Could you check a few things on this model? Use its own coordinates, in mm. A direction names the side the tool comes from. Give positions to 0.01 mm unless a question says otherwise; leave off trailing zeros. Order: outer loops, then holes, each group sorted by start corner. A loop starts at its lowest first (then second) coordinate and runs counter-clockwise, first axis right, second up. Notation, with made-up numbers: (-22.75, 12) -> (25.25, 12) arc R31 ccw to (25.25, 49) -> close; hole circle Ø4 at (-7.75, 56.25). An arc over 180 degrees is marked (long way). One line per item, written item: value.
```python
from build123d import *

# Parameters (mm, degrees)
SKETCH_1_W          = 15.8
SKETCH_1_H          = 127.8
EXTRUDE_1_DEPTH     = 3.2
SKETCH_2_R          = 2.4
EXTRUDE_2_DEPTH     = 1.7
SKETCH_3_R          = 2.5
CUT_EXTRUDE_1_DEPTH = 1.8


with BuildPart() as part:
    # Эскиз1 → Бобышка-Вытянуть1 (new body)
    with BuildSketch(Plane.XY):
        Rectangle(SKETCH_1_W, SKETCH_1_H)
    extrude(amount=EXTRUDE_1_DEPTH)

    # Эскиз2 → Бобышка-Вытянуть2 (add)
    with BuildSketch(Plane.XY.offset(3.2)):
        with Locations(Location((-4, 60, 0), (0, 0, 180))):
            Circle(SKETCH_2_R)
        with Locations(Location((4, 60, 0), (0, 0, 180))):
            Circle(SKETCH_2_R)
        with Locations(Location((4, 52, 0), (0, 0, 180))):
            Circle(SKETCH_2_R)
        with Locations(Location((4, 44, 0), (0, 0, 180))):
            Circle(SKETCH_2_R)
        with Locations(Location((4, 36, 0), (0, 0, 180))):
            Circle(SKETCH_2_R)
        with Locations(Location((4, 28, 0), (0, 0, 180))):
            Circle(SKETCH_2_R)
        with Locations(Location((4, 20, 0), (0, 0, 180))):
            Circle(SKETCH_2_R)
        with Locations(Location((4, 12, 0), (0, 0, 180))):
            Circle(SKETCH_2_R)
        with Locations(Location((4, 4, 0), (0, 0, 180))):
            Circle(SKETCH_2_R)
        with Locations(Location((4, -4, 0), (0, 0, 180))):
            Circle(SKETCH_2_R)
        with Locations(Location((4, -12, 0), (0, 0, 180))):
            Circle(SKETCH_2_R)
        with Locations(Location((4, -20, 0), (0, 0, 180))):
            Circle(SKETCH_2_R)
        with Locations(Location((4, -28, 0), (0, 0, 180))):
            Circle(SKETCH_2_R)
        with Locations(Location((4, -36, 0), (0, 0, 180))):
            Circle(SKETCH_2_R)
        with Locations(Location((4, -44, 0), (0, 0, 180))):
            Circle(SKETCH_2_R)
        with Locations(Location((4, -52, 0), (0, 0, 180))):
            Circle(SKETCH_2_R)
        with Locations(Location((4, -60, 0), (0, 0, 180))):
            Circle(SKETCH_2_R)
        with Locations(Location((-4, 52, 0), (0, 0, 180))):
            Circle(SKETCH_2_R)
        with Locations(Location((-4, 44, 0), (0, 0, 180))):
            Circle(SKETCH_2_R)
        with Locations(Location((-4, 36, 0), (0, 0, 180))):
            Circle(SKETCH_2_R)
        with Locations(Location((-4, 28, 0), (0, 0, 180))):
            Circle(SKETCH_2_R)
        with Locations(Location((-4, 20, 0), (0, 0, 180))):
            Circle(SKETCH_2_R)
        with Locations(Location((-4, 12, 0), (0, 0, 180))):
            Circle(SKETCH_2_R)
        with Locations(Location((-4, 4, 0), (0, 0, 180))):
            Circle(SKETCH_2_R)
        with Locations(Location((-4, -4, 0), (0, 0, 180))):
            Circle(SKETCH_2_R)
        with Locations(Location((-4, -12, 0), (0, 0, 180))):
            Circle(SKETCH_2_R)
        with Locations(Location((-4, -20, 0), (0, 0, 180))):
            Circle(SKETCH_2_R)
        with Locations(Location((-4, -28, 0), (0, 0, 180))):
            Circle(SKETCH_2_R)
        with Locations(Location((-4, -36, 0), (0, 0, 180))):
            Circle(SKETCH_2_R)
        with Locations(Location((-4, -44, 0), (0, 0, 180))):
            Circle(SKETCH_2_R)
        with Locations(Location((-4, -52, 0), (0, 0, 180))):
            Circle(SKETCH_2_R)
        with Locations(Location((-4, -60, 0), (0, 0, 180))):
            Circle(SKETCH_2_R)
    extrude(amount=EXTRUDE_2_DEPTH)

    # Эскиз3 → Вырез-Вытянуть1 (cut)
    with BuildSketch(Plane(origin=(0, 0, 0), x_dir=(-1, 0, 0), z_dir=(0, 0, -1))):
        with Locations((-4, 60)):
            Circle(SKETCH_3_R)
        with Locations((4, 60)):
            Circle(SKETCH_3_R)
        with Locations((4, 52)):
            Circle(SKETCH_3_R)
        with Locations((4, 44)):
            Circle(SKETCH_3_R)
        with Locations((4, 36)):
            Circle(SKETCH_3_R)
        with Locations((4, 28)):
            Circle(SKETCH_3_R)
        with Locations((4, 20)):
            Circle(SKETCH_3_R)
        with Locations((4, 12)):
            Circle(SKETCH_3_R)
        with Locations((4, 4)):
            Circle(SKETCH_3_R)
        with Locations((4, -4)):
            Circle(SKETCH_3_R)
        with Locations((4, -12)):
            Circle(SKETCH_3_R)
        with Locations((4, -20)):
            Circle(SKETCH_3_R)
        with Locations((4, -28)):
            Circle(SKETCH_3_R)
        with Locations((4, -36)):
            Circle(SKETCH_3_R)
        with Locations((4, -44)):
            Circle(SKETCH_3_R)
        with Locations((4, -52)):
            Circle(SKETCH_3_R)
        with Locations((4, -60)):
            Circle(SKETCH_3_R)
        with Locations((-4, 52)):
            Circle(SKETCH_3_R)
        with Locations((-4, 44)):
            Circle(SKETCH_3_R)
        with Locations((-4, 36)):
            Circle(SKETCH_3_R)
        with Locations((-4, 28)):
            Circle(SKETCH_3_R)
        with Locations((-4, 20)):
            Circle(SKETCH_3_R)
        with Locations((-4, 12)):
            Circle(SKETCH_3_R)
        with Locations((-4, 4)):
            Circle(SKETCH_3_R)
        with Locations((-4, -4)):
            Circle(SKETCH_3_R)
        with Locations((-4, -12)):
            Circle(SKETCH_3_R)
        with Locations((-4, -20)):
            Circle(SKETCH_3_R)
        with Locations((-4, -28)):
            Circle(SKETCH_3_R)
        with Locations((-4, -36)):
            Circle(SKETCH_3_R)
        with Locations((-4, -44)):
            Circle(SKETCH_3_R)
        with Locations((-4, -52)):
            Circle(SKETCH_3_R)
        with Locations((-4, -60)):
            Circle(SKETCH_3_R)
    extrude(amount=-CUT_EXTRUDE_1_DEPTH, mode=Mode.SUBTRACT)


solid = part.part
```
1) We'd pull the mould along X, two halves only. Please class faces 4 (the cylindrical face through (2.89, 38.13, 4.04)), 5 (the flat face through (-4, -44, 4.9)), 6 (the flat face through (-7.9, -1, 2)): +X half, -X half, draft (parallel to the pull), parting line (faces both ways), or undercut.
Answer below:
face 4: undercut
face 5: draft
face 6: -X half
2) If I drill on line 1 along X through (y, z) = (36, 3.5); line 2 along Z through (x, y) = (-2.25, 24); line 3 along Z through (x, y) = (-3, -11), over which ranges is the centre line in solid material (lowest first)?
Answer below:
line 1: x = -6.4 to -1.6, 1.6 to 6.4
line 2: z = 0 to 3.2
line 3: z = 1.8 to 4.9
3) For faces 1 (the flat face through (-4, -4, 1.8)), 2 (the flat face through (-4, 36, 4.9)), 3 (the cylindrical face through (-5.11, -33.87, 4.04)), which set-ups out of +Z, -Z, +X, -X, +Y, -Y let a thin tool reach every point of the face, with its end or its side?
Answer below:
face 1: -Z
face 2: +Z, +X, -X, +Y, -Y
face 3: +Z
4) For P1, Ø2.5, axis at x = -4, y = -53, coming from the -Z side; P2, Ø2, axis at y = 47.5, z = 4.5, coming from the -X side, each with a flat end and sliding along its axis, tell me the tip position at first contact or that it passes through.
Answer below:
P1: stops at z = 1.8
P2: passes through
5) Suppose I cut it at A-A, the plane y = -52. Write out the boundary of the cut face in (x, z).
Answer below:
outline: (-7.9, 0) -> (-6.5, 0) -> (-6.5, 1.8) -> (-1.5, 1.8) -> (-1.5, 0) -> (1.5, 0) -> (1.5, 1.8) -> (6.5, 1.8) -> (6.5, 0) -> (7.9, 0) -> (7.9, 3.2) -> (6.4, 3.2) -> (6.4, 4.9) -> (1.6, 4.9) -> (1.6, 3.2) -> (-1.6, 3.2) -> (-1.6, 4.9) -> (-6.4, 4.9) -> (-6.4, 3.2) -> (-7.9, 3.2) -> close
